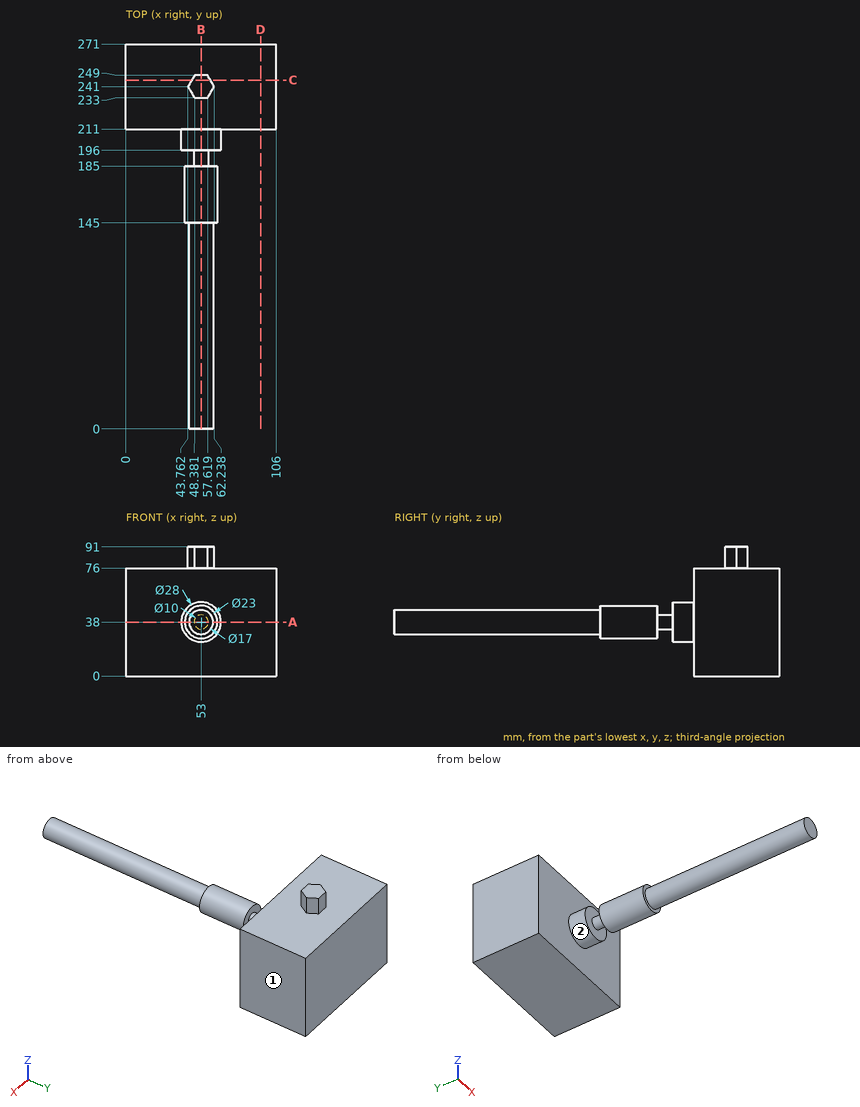
The drawing under review shows one solid part. Ordinate dimensions are in mm from its lowest x, y, z. A direction names the side the tool comes from. Coordinates: 2 decimals unless noted, no trailing zeros. Order: outer loops, then holes, each group sorted by start corner. A loop starts at its lowest first (then second) coordinate and runs counter-clockwise, first axis right, second up. Notation, with made-up numbers: M 29.5,74.5 L 83.5,74.5 A9 ccw 83.5,87.5 Z; hole C 6,-16.5 d2. An arc over 180 degrees is marked long. Use a Markdown table: item, result.
(1) Add section B-B (x = 53). Give the boundary of the cut face in (y, z).
Worked answers:
| item | result |
|---|---|
| outline | M 0,29.5 L 145,29.5 L 145,26.5 L 185,26.5 L 185,33 L 196,33 L 196,24 L 211,24 L 211,0 L 271,0 L 271,76 L 249,76 L 249,91 L 233,91 L 233,76 L 211,76 L 211,52 L 196,52 L 196,43 L 185,43 L 185,49.5 L 145,49.5 L 145,46.5 L 0,46.5 Z |
(2) Add section A-A (z = 38). Give the boundary of the cut face in (x, y), then the cut area to 3 significant figures.
Worked answers:
| item | result |
|---|---|
| outline | M 0,211 L 39,211 L 39,196 L 48,196 L 48,185 L 41.5,185 L 41.5,145 L 44.5,145 L 44.5,0 L 61.5,0 L 61.5,145 L 64.5,145 L 64.5,185 L 58,185 L 58,196 L 67,196 L 67,211 L 106,211 L 106,271 L 0,271 Z |
| area | 10,300 mm2 |
(3) Add section D-D (x = 95). Give the boundary of the cut face in (y, z), then the cut area to 3 significant figures.
Worked answers:
| item | result |
|---|---|
| outline | M 211,0 L 271,0 L 271,76 L 211,76 Z |
| area | 4,560 mm2 |
(4) For the marked faces 1 and 2, list the 3-axis set-ups (+Z, -Z, +X, -X, +Y, -Y) from which the entire face can be reached by the end or side of a thin tool; tool diameter is ignored.
Worked answers:
| item | result |
|---|---|
| face 1 | +Z, -Z, +X, +Y, -Y |
| face 2 | -Y |
(5) For P1, Ø4, axis at x = 56.5, y = 227.5, coming from the +Z side; P2, Ø4.5, axis at x = 55, z = 82, coming from the +Y side; P3, Ø4.5, axis at x = 52, z = 87, coming from the -Y side, all flat-tipped, find the tip position at first contact; note any pin that passes through.
Worked answers:
| item | result |
|---|---|
| P1 | stops at z = 76 |
| P2 | stops at y = 249 |
| P3 | stops at y = 233 |
(6) Wall thickness on probe 1 along Y at (x, z) = (26, 37.5); probe 2 along X at (y, z) = (151, 37); probe 3 along Z at (x, y) = (35.5, 254): over which ranges is each line inside the solid? List them lowest first.
Worked answers:
| item | result |
|---|---|
| probe 1 | y = 211 to 271 |
| probe 2 | x = 41.54 to 64.46 |
| probe 3 | z = 0 to 76 |
(7) Add section C-C (y = 245.5). Give the boundary of the cut face in (x, z).
Worked answers:
| item | result |
|---|---|
| outline | M 0,0 L 106,0 L 106,76 L 59.64,76 L 59.64,91 L 46.36,91 L 46.36,76 L 0,76 Z |
